```python
from build123d import *

# Parameters (mm, degrees)
SKETCH_1_W                      = 100
SKETCH_1_H                      = 50
EXTRUDE_1_DEPTH                 = 10
HOLE_WIZARD_5_0_5_1_D           = 5
HOLE_WIZARD_5_0_5_1_CSINK_D     = 5.05
HOLE_WIZARD_5_0_5_1_CSINK_ANGLE = 90
SKETCH_20_R                     = 5
CUT_EXTRUDE_1_DEPTH             = 57.789083458
SKETCH_26_R                     = 12.5
CUT_EXTRUDE_2_DEPTH             = 2.5
HOLE_WIZARD_M3_1_D              = 2.5
HOLE_WIZARD_M3_1_CSINK_D        = 3.05
HOLE_WIZARD_M3_1_CSINK_ANGLE    = 90
SKETCH_35_R                     = 12.5
CUT_EXTRUDE_3_DEPTH             = 57.402570863


with BuildPart() as part:
    # 草图1 → 凸台-拉伸1 (new body)
    with BuildSketch(Plane.XY):
        Rectangle(SKETCH_1_W, SKETCH_1_H)
    extrude(amount=EXTRUDE_1_DEPTH)

    # Ø5.0 (5) 直径孔1 (through all)
    with Locations(Plane.XY.offset(10)):
        with Locations((0, 18), (0, -18)):
            CounterSinkHole(HOLE_WIZARD_5_0_5_1_D / 2, HOLE_WIZARD_5_0_5_1_CSINK_D / 2, counter_sink_angle=HOLE_WIZARD_5_0_5_1_CSINK_ANGLE)

    # 草图20 → 切除-拉伸1 (cut, through all)
    with BuildSketch(Plane.XY.offset(10)):
        Circle(SKETCH_20_R)
    extrude(amount=-CUT_EXTRUDE_1_DEPTH, mode=Mode.SUBTRACT)

    # 草图25 → Ø8.2 (8.2) 直径孔1 (revolve, cut)
    with BuildSketch(Plane(origin=(30, 0, 10), x_dir=(0, -1, 0), z_dir=(1, 0, 0))):
        Polygon((0, 0), (0, 10), (4.125, 10), (4.1, 9.975), (4.1, 0.025), (4.125, 0), align=None)
    hole_wizard_8_2_8_2_1 = revolve(axis=Axis((30, 0, 16.35), (0, 0, -1)), mode=Mode.SUBTRACT)

    # 镜向1: Ø8.2 (8.2) 直径孔1 across plane
    add(hole_wizard_8_2_8_2_1.mirror(Plane(origin=(0, 0, 0), x_dir=(0, 0, 1), z_dir=(1, 0, 0))), mode=Mode.SUBTRACT)

    # 草图26 → 切除-拉伸2 (cut)
    with BuildSketch(Plane(origin=(0, 0, 0), x_dir=(-1, 0, 0), z_dir=(0, 0, -1))):
        Circle(SKETCH_26_R)
    extrude(amount=-CUT_EXTRUDE_2_DEPTH, mode=Mode.SUBTRACT)

    # M3 螺纹孔1 (through all)
    with Locations(Plane.XY.offset(10)):
        with Locations((15.565692097, 15.434028299), (15.434028299, -15.565692097), (-15.565692097, -15.434028299), (-15.434028299, 15.565692097)):
            CounterSinkHole(HOLE_WIZARD_M3_1_D / 2, HOLE_WIZARD_M3_1_CSINK_D / 2, counter_sink_angle=HOLE_WIZARD_M3_1_CSINK_ANGLE)

    # 草图35 → 切除-拉伸3 (cut, through all)
    with BuildSketch(Plane(origin=(0, 0, 2.5), x_dir=(-1, 0, 0), z_dir=(0, 0, -1))):
        Circle(SKETCH_35_R)
    extrude(amount=-CUT_EXTRUDE_3_DEPTH, mode=Mode.SUBTRACT)


solid = part.part
```
CAD build for the part. Positions are in the model's coordinates, mm. Give positions to 0.01 mm unless a question says otherwise; leave off trailing zeros. Loops run counter-clockwise (first coordinate to the right, second up) from the corner with the lowest first, then second, coordinate; pieces in that order, holes last. Notation, with made-up numbers: M 64,-10 L 116,-10 A11 ccw 116,-4 Z; hole C 14,63.5 d6. An arc over 180 degrees is marked long. Use one line per item in the form item = value.
Item 1: Slice it at D-D (z = 4.25). Count the separate pieces of the cut face and the enclosed holes in it, plus the area to 3 significant figures.
Determined:
separate_pieces = 1
enclosed_holes = 9
area = 4,340 mm2
Item 2: Two-plate mould, pull along X, no slides. Class faces 1 (the face through (-1, -25, 5)), 2 (the face through (50, 0, 5)), 3 (the face through (-11.923, 3.755, 4.93)): pulls with the +X half, pulls with the -X half, needs draft (parallel to the pull), parting line crosses it, or undercut.
Determined:
face_1 = needs draft
face_2 = pulls with the +X half
face_3 = undercut
Item 3: Drill centre lines: probe 1 along Y at (x, z) = (0, 4.25); probe 2 along X at (y, z) = (1.5, 5); probe 3 along X at (y, z) = (2, 1.5). Where is each one in solid material? Low to high. Write a range as from..to.
Determined:
probe_1 = -25..-20.5, -15.5..-12.5, 12.5..15.5, 20.5..25
probe_2 = -50..-33.82, -26.18..-12.41, 12.41..26.18, 33.82..50
probe_3 = -50..-33.58, -26.42..-12.34, 12.34..26.42, 33.58..50
Item 4: Slice it at A-A (x = 0). List the corners of the cut face in (y, z) (3 decimals), plus the area to 3 significant figures.
Determined:
outline = M -25,0 L -20.5,0 L -20.5,9.975 L -20.525,10 L -25,10 Z; M -15.5,0 L -12.5,0 L -12.5,10 L -15.475,10 L -15.5,9.975 Z; M 12.5,0 L 15.5,0 L 15.5,9.975 L 15.475,10 L 12.5,10 Z; M 20.5,0 L 25,0 L 25,10 L 20.525,10 L 20.5,9.975 Z
area = 150 mm2
Item 5: Slice it at B-B (x = -30). List the corners of the cut face in (y, z) (3 decimals), plus the area to 3 significant figures.
Determined:
outline = M -25,0 L -4.125,0 L -4.1,0.025 L -4.1,9.975 L -4.125,10 L -25,10 Z; M 4.1,0.025 L 4.125,0 L 25,0 L 25,10 L 4.125,10 L 4.1,9.975 Z
area = 418 mm2
Item 6: Slice it at C-C (y = -18). List the corners of the cut face in (x, z) (3 decimals).
Determined:
outline = M -50,0 L -2.5,0 L -2.5,9.975 L -2.525,10 L -50,10 Z; M 2.5,0 L 50,0 L 50,10 L 2.525,10 L 2.5,9.975 Z
